Autodesk Inventor part; units mm, degrees
ref_plane "YZ Plane" through (0, 0, 0) normal (1, 0, 0) x (0, 1, 0)
ref_plane "XZ Plane" through (0, 0, 0) normal (0, 1, 0) x (-1, 0, 0)
ref_plane "XY Plane" through (0, 0, 0) normal (0, 0, 1) x (1, 0, 0)
sketch "Esquisse1" plane through (0, 0, 0) normal (0, 1, 0) x (-1, 0, 0)
  line L0 (-30, 25) -> (30, 25)
  line L1 (30, 25) -> (30, -40)
  line L2 (30, -40) -> (-30, -40)
  line L3 (-30, -40) -> (-30, 25)
  line L4 (-30, 25) -> (-70, 25) construction
  line L5 (-70, 25) -> (-70, 0) construction
  line L6 (-70, 0) -> (-30, 0) construction
  line L7 (-30, 0) -> (-30, 25) construction
  line L8 (30, 25) -> (70, 25) construction
  line L9 (70, 25) -> (70, 0) construction
  line L10 (70, 0) -> (30, 0) construction
  line L11 (30, 0) -> (30, 25) construction
  line L12 (-50, 0) -> (50, 0) construction
  line L13 (50, 0) -> (50, -40) construction
  line L14 (50, -40) -> (-50, -40) construction
  line L15 (-50, -40) -> (-50, 0) construction
  circle A0 centre (-50, 0) radius 20
  circle A1 centre (50, 0) radius 20
  line L16 (-70, 0) -> (-30, 25)
  line L17 (70, 0) -> (30, 25)
  line L18 (50, -20) -> (-50, -20)
  line L19 (-70, 0) -> (-50, -20)
  line L20 (50, -20) -> (70, 0)
  point P0 (0, 0)
  dimension "d8" = 40
  dimension "d9" = 40
  dimension "d0" = 25
  dimension "d1" = 140
  dimension "d2" = 60
  dimension "d3" = 65
  dimension "d4" = 30
  dimension "d5" = 25
  dimension "d6" = 100
  dimension "d7" = 50
  dimension "d10" = 70
extrude "Extrusion1" add sketch "Esquisse1" along normal blind 5
sketch "Esquisse2" plane through (0, 5, 0) normal (0, 1, 0) x (1, 0, 0)
  arc A0 (41.236, -17.9775) -> (50, 20) centre (50, 0) ccw
  arc A1 (-50, 20) -> (-41.236, -17.9775) centre (-50, 0) ccw
  circle A2 centre (-50, 0) radius 3
  circle A3 centre (50, 0) radius 3
  point P0 (0, 0)
  dimension "d13" = 6
  dimension "d14" = 6
extrude "Extrusion2" cut sketch "Esquisse2" against normal through all
sketch "Esquisse3" plane through (0, 5, 0) normal (0, 1, 0) x (1, 0, 0)
  circle A0 centre (-50, 0) radius 3
  circle A1 centre (50, 0) radius 3
  line L0 (30, 40) -> (-30, 40)
  arc A2 (-50, 20) -> (-41.236, -17.9775) centre (-50, 0) ccw
  line L1 (0, 0) -> (0, 40) construction
  line L2 (-50, 0) -> (-50, 20) construction
  circle A3 centre (-50, 0) radius 15 construction
  circle A4 centre (-50, 15) radius 4.5
  circle A5 centre (50, 15) radius 4.5
  circle A6 centre (-60.6066, 10.6066) radius 4.5
  circle A7 centre (-65, 0) radius 4.5
  circle A8 centre (-60.6066, -10.6066) radius 4.5
  circle A9 centre (-50, -15) radius 4.5
  circle A10 centre (-39.3934, -10.6066) radius 4.5
  circle A11 centre (-35, 0) radius 4.5
  circle A12 centre (-39.3934, 10.6066) radius 4.5
  circle A13 centre (39.3934, 10.6066) radius 4.5
  circle A14 centre (35, 0) radius 4.5
  circle A15 centre (39.3934, -10.6066) radius 4.5
  circle A16 centre (50, -15) radius 4.5
  circle A17 centre (60.6066, -10.6066) radius 4.5
  circle A18 centre (65, 0) radius 4.5
  circle A19 centre (60.6066, 10.6066) radius 4.5
  dimension "d17" = 30
  dimension "d18" = 9
  dimension "d21" = 360
  dimension "d25" = 360
extrude "Extrusion3" cut sketch "Esquisse3" against normal blind 2.5 contours A4 | A5 | A6 | A7 | A8 | A9 | A10 | A11 | A12 | A13 | A14 | A15 | A16 | A17 | A18 | A19
equation "\"d9\" = d8"
equation "\"d14\" = d13"
properties part number "support_puissance"
Geometry check sheet. Reference: the model listing, model coordinates, mm. A direction names the side the tool comes from. Round coordinates to 2 decimals unless told otherwise and drop trailing zeros. Order: outer loops, then holes, each group sorted by start corner. A loop starts at its lowest first (then second) coordinate and runs counter-clockwise, first axis right, second up. Notation, with made-up numbers: (-40, -28) - (3, -28) arc R19 ccw to (3, -24) - close; hole circle Ø2 at (38, 21.25). An arc over 180 degrees is marked (long way). One line per question, with ' | ' between items. Start each with the question number.
(1) Access from +Z, -Z, +X, -X, +Y, -Y to the whole of each face (thin tool, end or side, straight path). Record for faces 4 (the flat face through (-35.697, 2.465, 21.44)), 5 (the flat face through (0, 2, 25)), 6 (the flat face through (61, 2.5, 11)).
(2) Sectioned sample at D-D on z = -24. Record the cut outline in (x, y), and give its area (3 significant figures).
(3) Release check for a two-part mould opening along Z. For faces 1 (the flat face through (1, 0, 0)), 2 (the flat face through (35.697, 2.465, 21.44)), 3 (the cylindrical face through (64.899, 3.768, 9.255)) record: released by +Z, released by -Z, zero draft, split by the parting line, or undercut.
(4) Sectioned sample at A-A on y = 3.3. Count the separate pieces of the cut face and the enclosed holes in it, and give its area (3 significant figures).
(5) Depth check by flat-ended pin: pin 1 Ø1 at (y, z) = (2, 7.5) entering from +X (3 decimals); pin 2 Ø8 at (x, z) = (39.39, 10.61) entering from +Y; pin 3 Ø2.5 at (y, z) = (2, -35) entering from +X; pin 4 Ø3.5 at (x, z) = (50, 0) entering from +Y. Enter the tip coordinate at first touch or a pass-through.
(6) Sectioned sample at C-C on x = -32. Record the cut outline in (y, z), and give its area (3 significant figures).
(7) Sectioned sample at B-B on z = 13. Record the cut outline in (x, y).
(8) Thickness scan on L1, parallel to Z at x = 50, y = 3.75; L2, parallel to X at y = 3.75, z = -6.5; L3, parallel to Z at x = 59.5, y = 3.75. Record the ranges inside material, lowest first. Write a range as [from, to].
Conclusion:
1) face 4: +Z, +Y, -Y | face 5: +Z, +X, -X, +Y, -Y | face 6: +Y
2) outline: (-30, 0) - (30, 0) - (30, 5) - (-30, 5) - close | area: 300 mm2
3) face 1: zero draft | face 2: released by +Z | face 3: undercut
4) separate pieces: 1 | enclosed holes: 18 | area: 5,700 mm2
5) pin 1: stops at x = 68.735 | pin 2: stops at y = 2.5 | pin 3: stops at x = 30 | pin 4: passes through
6) outline: (0, -20) - (5, -20) - (5, -3.35) - (2.5, -3.35) - (2.5, 3.35) - (5, 3.35) - (5, 23.75) - (0, 23.75) - close | area: 202 mm2
7) outline: (-65.2, 0) - (65.2, 0) - (65.2, 5) - (64.42, 5) - (64.42, 2.5) - (56.8, 2.5) - (56.8, 5) - (54.03, 5) - (54.03, 2.5) - (45.97, 2.5) - (45.97, 5) - (43.2, 5) - (43.2, 2.5) - (35.58, 2.5) - (35.58, 5) - (-35.58, 5) - (-35.58, 2.5) - (-43.2, 2.5) - (-43.2, 5) - (-45.97, 5) - (-45.97, 2.5) - (-54.03, 2.5) - (-54.03, 5) - (-56.8, 5) - (-56.8, 2.5) - (-64.42, 2.5) - (-64.42, 5) - (-65.2, 5) - close
8) L1: z = [-20, -19.5], [-10.5, -3], [3, 10.5], [19.5, 20] | L2: x = [-68.91, -62.45], [-58.77, -41.23], [-37.55, 37.55], [41.23, 58.77], [62.45, 68.91] | L3: z = [-17.6, -14.97], [-6.24, 6.24], [14.97, 17.6]
